Design review of the part shown in the three views and the two pictorial views. Dimensions are in mm from the part's minimum x, y and z. A direction names the side the tool comes from. Give positions to 0.01 mm unless a question says otherwise; leave off trailing zeros. Order: outer loops, then holes, each group sorted by start corner. A loop starts at its lowest first (then second) coordinate and runs counter-clockwise, first axis right, second up.
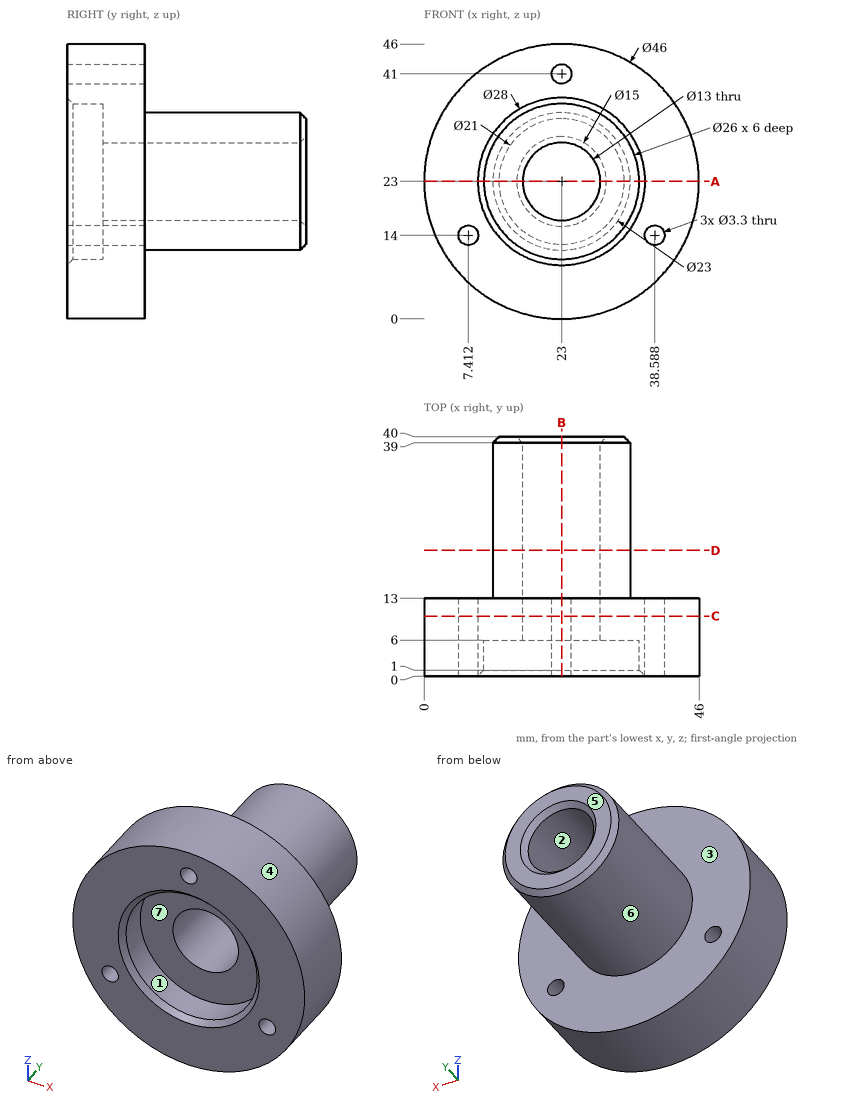
Item 1: Clearance check with flat-ended pins moving along their axes: pin 1 Ø5.5 at (x, z) = (23, 41) entering from +Y; pin 2 Ø2 at (x, y) = (30, 12) entering from -Z; pin 3 Ø4 at (y, z) = (20.5, 33.5) entering from +X (1 decimal). State where each tip first meets the part, or that it passes through.
Values found:
pin 1: stops at y = 13
pin 2: stops at z = 0.8
pin 3: stops at x = 30.7
Item 2: For line 1 (Z direction, x = 23, y = 2.45); line 2 (Z direction, x = 23, y = 10.25); line 3 (X direction, y = 23.5, z = 23), list the stretches that pass through material, from the lowest coordinate up.
Values found:
line 1: z = 0 to 10, 36 to 39.35, 42.65 to 46
line 2: z = 0 to 16.5, 29.5 to 39.35, 42.65 to 46
line 3: x = 11.5 to 16.5, 29.5 to 34.5
Item 3: For the marked faces 5, 6 and 7, list the 3-axis set-ups (+Z, -Z, +X, -X, +Y, -Y) from which the entire face can be reached by the end or side of a thin tool; tool diameter is ignored.
Values found:
face 5: +Z, -Z, +X, -X, +Y
face 6: +Y
face 7: -Y
Item 4: Take a section at B-B (x = 23). Give the boundary of the cut face in (y, z).
Values found:
outline: (0, 0) - (13, 0) - (13, 11.5) - (39, 11.5) - (40, 12.5) - (40, 15.5) - (39, 16.5) - (6, 16.5) - (6, 10) - (1, 10) - (0, 9) - close; (0, 37) - (1, 36) - (6, 36) - (6, 29.5) - (39, 29.5) - (40, 30.5) - (40, 33.5) - (39, 34.5) - (13, 34.5) - (13, 39.35) - (0, 39.35) - close; (0, 42.65) - (13, 42.65) - (13, 46) - (0, 46) - close
Item 5: Take a section at C-C (y = 10). Give the boundary of the cut face in (x, z).
Values found:
outline: circle Ø46 at (23, 23); hole circle Ø3.3 at (7.41, 14); hole circle Ø13 at (23, 23); hole circle Ø3.3 at (23, 41); hole circle Ø3.3 at (38.59, 14)
Item 6: Take a section at D-D (y = 21). Give the boundary of the cut face in (x, z), and give its area (3 significant figures).
Values found:
outline: circle Ø23 at (23, 23); hole circle Ø13 at (23, 23)
area: 283 mm2
Item 7: Take a section at A-A (z = 23). Give the boundary of the cut face in (x, y).
Values found:
outline: (0, 0) - (9, 0) - (10, 1) - (10, 6) - (16.5, 6) - (16.5, 39) - (15.5, 40) - (12.5, 40) - (11.5, 39) - (11.5, 13) - (0, 13) - close; (29.5, 6) - (36, 6) - (36, 1) - (37, 0) - (46, 0) - (46, 13) - (34.5, 13) - (34.5, 39) - (33.5, 40) - (30.5, 40) - (29.5, 39) - close
Item 8: Draft analysis for pull direction X (two halves, no side actions). For the marked faces 1, 2, 3 and 4, state which applies: released by +X, released by -X, zero draft, split by the parting line, or undercut.
Values found:
face 1: undercut
face 2: undercut
face 3: zero draft
face 4: split by the parting line
